Could you check a few things on this model? Use its own coordinates, in mm. A direction names the side the tool comes from. Give positions to 0.01 mm unless a question says otherwise; leave off trailing zeros. Loops run counter-clockwise (first coordinate to the right, second up) from the corner with the lowest first, then second, coordinate; pieces in that order, holes last.
1. Imagine slicing it at D-D (z = 4.5). List the corners of the cut face in (x, y) for me, plus the area to 3 significant figures.
2. Imagine slicing it at A-A (y = 18). List the corners of the cut face in (x, z) for me.
3. Imagine slicing it at C-C (y = -227). List the corners of the cut face in (x, z) for me.
4. For P1, Ø9.5, axis at x = 402.5, z = 13.5, coming from the -Y side; P2, Ø9.5, axis at y = -231.5, z = 9.5, coming from the -X side, each with a flat end and sliding along its axis, tell me the tip position at first contact or that it passes through.
5. I need wall thicknesses on line 1 along X through (y, z) = (-49.5, 13.5); line 2 along X through (y, z) = (110, 15.5); line 3 along Y through (x, z) = (327.5, 12). Which ranges of each line are inside material? Lowest first, please.
6. Imagine slicing it at B-B (x = 277). List the corners of the cut face in (y, z) for me, plus the area to 3 significant figures.
7. For faces 1 (the flat face through (304, 115.954, 9)), 2 (the flat face through (-355.6, -231, 9)), 3 (the flat face through (6, 175.796, 9)), 4 (the flat face through (-4, -205.204, 9)), 5 (the flat face through (355.6, -231, 9)), which set-ups out of +Z, -Z, +X, -X, +Y, -Y let a thin tool reach every point of the face, with its end or its side?
8. Thinking about a two-plate mould opening in X: for faces 6 (the flat face through (406, -205.204, 9)), 7 (the flat face through (-457.2, -12, 9)), 8 (the flat face through (-306, 115.954, 9)), which applies, +X half, -X half, draft (parallel to the pull), parting line (faces both ways), or undercut?
```python
from build123d import *

# Parameters (mm, degrees)
F0_W     = 101.6
F0_H     = 254
F0_H_2   = 50.8
F1_DEPTH = 19.05


with BuildPart() as f1:
    # F0 (on Top) → F1 (new body)
    with BuildSketch(Plane.XY):
        with BuildLine():
            ThreePointArc((12.70004, -50.177005), (-8.980216, -41.196749), (4e-05, -62.877005))
            ThreePointArc((4e-05, -62.877005), (8.980296, -59.157261), (12.70004, -50.177005))
        make_face()
        Polygon((457.2, 175.795518), (-457.2, 175.795518), (-457.2, -205.204482), (-355.6, -205.204482), (-254, -205.204482), (4e-05, -205.204482), (254, -205.204482), (355.6, -205.204482), (457.2, -205.204482), align=None)
        with BuildLine():
            ThreePointArc((12.70004, -50.177005), (8.980296, -59.157261), (4e-05, -62.877005))
            ThreePointArc((4e-05, -62.877005), (-8.980216, -41.196749), (12.70004, -50.177005))
        make_face(mode=Mode.SUBTRACT)
        with Locations((-304.8, -11.045669)):
            Rectangle(F0_W, F0_H, mode=Mode.SUBTRACT)
        with Locations((304.8, -11.045669)):
            Rectangle(F0_W, F0_H, mode=Mode.SUBTRACT)
        with Locations((-304.8, -230.604482)):
            Rectangle(F0_W, F0_H_2)
        with Locations((304.8, -230.604482)):
            Rectangle(F0_W, F0_H_2)
    extrude(amount=F1_DEPTH)


solid = f1.part
```
Derived:
1. outline: (-457.2, -205.2) - (-355.6, -205.2) - (-355.6, -256) - (-254, -256) - (-254, -205.2) - (254, -205.2) - (254, -256) - (355.6, -256) - (355.6, -205.2) - (457.2, -205.2) - (457.2, 175.8) - (-457.2, 175.8) - close; hole (-355.6, -138.05) - (-254, -138.05) - (-254, 115.95) - (-355.6, 115.95) - close; hole circle Ø25.4 at (0, -50.18); hole (254, -138.05) - (355.6, -138.05) - (355.6, 115.95) - (254, 115.95) - close
1. area: 307,000 mm2
2. outline: (-457.2, 0) - (-355.6, 0) - (-355.6, 19.05) - (-457.2, 19.05) - close; (-254, 0) - (254, 0) - (254, 19.05) - (-254, 19.05) - close; (355.6, 0) - (457.2, 0) - (457.2, 19.05) - (355.6, 19.05) - close
3. outline: (-355.6, 0) - (-254, 0) - (-254, 19.05) - (-355.6, 19.05) - close; (254, 0) - (355.6, 0) - (355.6, 19.05) - (254, 19.05) - close
4. P1: stops at y = -205.2
4. P2: stops at x = -355.6
5. line 1: x = -457.2 to -355.6, -254 to -12.68, 12.68 to 254, 355.6 to 457.2
5. line 2: x = -457.2 to -355.6, -254 to 254, 355.6 to 457.2
5. line 3: y = -256 to -138.05, 115.95 to 175.8
6. outline: (-256, 0) - (-138.05, 0) - (-138.05, 19.05) - (-256, 19.05) - close; (115.95, 0) - (175.8, 0) - (175.8, 19.05) - (115.95, 19.05) - close
6. area: 3,390 mm2
7. face 1: +Z, -Z
7. face 2: +Z, -Z, -X, -Y
7. face 3: +Z, -Z, +X, -X, +Y
7. face 4: +Z, -Z, -Y
7. face 5: +Z, -Z, +X, -Y
8. face 6: draft
8. face 7: -X half
8. face 8: undercut
